Read the model definition and answer for the solid it produces. Units are mm, in the model's axes. A direction names the side the tool comes from. Coordinates: 2 decimals unless noted, no trailing zeros. Loops run counter-clockwise (first coordinate to the right, second up) from the corner with the lowest first, then second, coordinate; pieces in that order, holes last.
from build123d import *

# Parameters (mm, degrees)
SALIENTE_EXTRUIR1_DEPTH = 3
SALIENTE_EXTRUIR2_DEPTH = 1
CROQUIS1_7_W            = 1.8
CROQUIS1_7_H            = 10
SALIENTE_EXTRUIR4_DEPTH = 9.5
REDONDEO2_R             = 5
CROQUIS3_R              = 1.5
CORTAR_EXTRUIR2_DEPTH   = 16


with BuildPart() as part:
    # Croquis1 → Saliente-Extruir1 (new, symmetric)
    with BuildSketch(Plane(origin=(0, 0, 0), x_dir=(1, 0, 0), z_dir=(0, 1, 0))):
        with BuildLine():
            Line((-1.861867424, 4.190006044), (10.856046359, 4.190006044))
            ThreePointArc((10.856046359, 4.190006044), (12.977366702, 3.311326387), (13.856046359, 1.190006044))
            Line((13.856046359, 1.190006044), (13.856046359, -78.809993956))
            Line((13.856046359, -78.809993956), (10.856046359, -78.809993956))
            ThreePointArc((10.856046359, -78.809993956), (8.734726015, -77.9313143), (7.856046359, -75.809993956))
            Line((7.856046359, -75.809993956), (7.856046359, -40.566421369))
            Line((7.856046359, -40.566421369), (-4.195556186, -3.47994934))
            ThreePointArc((-4.195556186, -3.47994934), (-5.870430721, 1.219660174), (-1.861867424, 4.190006044))
        make_face()
        with BuildLine():
            Line((-1.861867424, 2.6), (2.138132576, 2.6))
            ThreePointArc((2.138132576, 2.6), (4.738132576, 0), (2.138132576, -2.6))
            Line((2.138132576, -2.6), (-1.861867424, -2.6))
            ThreePointArc((-1.861867424, -2.6), (-4.461867424, 0), (-1.861867424, 2.6))
        make_face(mode=Mode.SUBTRACT)
        Polygon((0.241081645, -4.190006044), (7.856046359, -4.190006044), (7.856046359, -27.623584675), align=None, mode=Mode.SUBTRACT)
    extrude(amount=SALIENTE_EXTRUIR1_DEPTH, both=True)

    # Croquis1<3> → Saliente-Extruir2 (add, symmetric)
    with BuildSketch(Plane(origin=(0, 0, 0), x_dir=(1, 0, 0), z_dir=(0, 1, 0))):
        with BuildLine():
            ThreePointArc((-1.861867424, 2.6), (-3.700345055, 1.838477631), (-4.461867424, 0))
            ThreePointArc((-4.461867424, 0), (-3.700345055, -1.838477631), (-1.861867424, -2.6))
            Line((-1.861867424, -2.6), (2.138132576, -2.6))
            ThreePointArc((2.138132576, -2.6), (4.738132576, 0), (2.138132576, 2.6))
            Line((2.138132576, 2.6), (-1.861867424, 2.6))
        make_face()
        with BuildLine():
            ThreePointArc((-0.591867424, 0), (-1.861867424, -1.27), (-3.131867424, 0))
            ThreePointArc((-3.131867424, 0), (-1.861867424, 1.27), (-0.591867424, 0))
        make_face(mode=Mode.SUBTRACT)
        with BuildLine():
            ThreePointArc((3.408132576, 0), (2.138132576, -1.27), (0.868132576, 0))
            ThreePointArc((0.868132576, 0), (2.138132576, 1.27), (3.408132576, 0))
        make_face(mode=Mode.SUBTRACT)
    extrude(amount=SALIENTE_EXTRUIR2_DEPTH, both=True)

    # Croquis1<7> → Saliente-Extruir4 (add, symmetric)
    with BuildSketch(Plane(origin=(0, 0, 0), x_dir=(1, 0, 0), z_dir=(0, 1, 0))):
        with Locations((12.956046359, -9.190006044)):
            Rectangle(CROQUIS1_7_W, CROQUIS1_7_H)
        with Locations((12.956046359, -69.190006044)):
            Rectangle(CROQUIS1_7_W, CROQUIS1_7_H)
    extrude(amount=SALIENTE_EXTRUIR4_DEPTH, both=True)

    # Redondeo2
    # the kernel refuses this fillet: 5 mm, written as the material it takes off along each edge
    with BuildSketch(Plane(origin=(-0.443953641, -9.5, 74.190006044), x_dir=(0, 1, 0), z_dir=(1, 0, 0)), Plane(origin=(26.356046359, -9.5, 64.190006044), x_dir=(0, 1, 0), z_dir=(-1, 0, 0)), Plane(origin=(-0.443953641, -9.5, 14.190006044), x_dir=(0, 1, 0), z_dir=(1, 0, 0)), Plane(origin=(26.356046359, -9.5, 4.190006044), x_dir=(0, 1, 0), z_dir=(-1, 0, 0))) as redondeo2_piece_1:
        with BuildLine():
            CenterArc((REDONDEO2_R, -REDONDEO2_R), REDONDEO2_R, 90, 90)
            Line((0, -REDONDEO2_R), (-REDONDEO2_R * 0.02, -REDONDEO2_R))
            Line((-REDONDEO2_R * 0.02, -REDONDEO2_R), (-REDONDEO2_R * 0.02, REDONDEO2_R * 0.02))
            Line((-REDONDEO2_R * 0.02, REDONDEO2_R * 0.02), (REDONDEO2_R, REDONDEO2_R * 0.02))
            Line((REDONDEO2_R, REDONDEO2_R * 0.02), (REDONDEO2_R, 0))
        make_face()
    extrude(amount=26.8, mode=Mode.SUBTRACT)
    with BuildSketch(Plane(origin=(-0.443953641, 9.5, 74.190006044), x_dir=(0, -1, 0), z_dir=(1, 0, 0)), Plane(origin=(26.356046359, 9.5, 64.190006044), x_dir=(0, -1, 0), z_dir=(-1, 0, 0)), Plane(origin=(-0.443953641, 9.5, 14.190006044), x_dir=(0, -1, 0), z_dir=(1, 0, 0)), Plane(origin=(26.356046359, 9.5, 4.190006044), x_dir=(0, -1, 0), z_dir=(-1, 0, 0))) as redondeo2_piece_2:
        with BuildLine():
            CenterArc((REDONDEO2_R, REDONDEO2_R), REDONDEO2_R, 180, 90)
            Line((0, REDONDEO2_R), (-REDONDEO2_R * 0.02, REDONDEO2_R))
            Line((-REDONDEO2_R * 0.02, REDONDEO2_R), (-REDONDEO2_R * 0.02, -REDONDEO2_R * 0.02))
            Line((-REDONDEO2_R * 0.02, -REDONDEO2_R * 0.02), (REDONDEO2_R, -REDONDEO2_R * 0.02))
            Line((REDONDEO2_R, -REDONDEO2_R * 0.02), (REDONDEO2_R, 0))
        make_face()
    extrude(amount=26.8, mode=Mode.SUBTRACT)

    # Croquis3 → Cortar-Extruir2 (cut)
    with BuildSketch(Plane(origin=(13.856046359, 0, 0), x_dir=(0, 0, -1), z_dir=(1, 0, 0))):
        with Locations((-69.190006044, 7.5)):
            Circle(CROQUIS3_R)
        with Locations((-69.190006044, -7.5)):
            Circle(CROQUIS3_R)
        with Locations((-9.190006044, 7.5)):
            Circle(CROQUIS3_R)
        with Locations((-9.190006044, -7.5)):
            Circle(CROQUIS3_R)
    extrude(amount=-CORTAR_EXTRUIR2_DEPTH, mode=Mode.SUBTRACT)


solid = part.part
Item 1: A cutting plane is placed at C-C on y = 2. Determine the outline of the cut face in (x, z), then the cut area to 3 significant figures.
Numbers:
outline: (-4.2, 3.48) arc R4.19 ccw to (-1.86, -4.19) - (10.86, -4.19) arc R3 ccw to (13.86, -1.19) - (13.86, 78.81) - (10.86, 78.81) arc R3 ccw to (7.86, 75.81) - (7.86, 40.57) - close; hole (-1.86, -2.6) - (2.14, -2.6) arc R2.6 ccw to (2.14, 2.6) - (-1.86, 2.6) arc R2.6 ccw to start; hole (0.24, 4.19) - (7.86, 4.19) - (7.86, 27.62) - close
area: 687 mm2
Item 2: Which of the six approach directions +Z, -Z, +X, -X, +Y, -Y give full straight-line access (tool end or side, diameter ignored) to faces 5 (the face through (4, 0, 4.19)), 6 (the face through (4.738, 2.014, -0.057)), 7 (the face through (13, -4, 4.19)), 8 (the face through (4.738, -1.986, -0.057))?
Numbers:
face 5: +Y, -Y
face 6: +Y
face 7: -Z, +X, -X, -Y
face 8: -Y
Item 3: A cutting plane is placed at A-A on z = 0. Determine the outline of the cut face in (x, y).
Numbers:
outline: (-6.05, -3) - (-4.46, -3) - (-4.46, -1) - (-3.13, -1) - (-3.13, 1) - (-4.46, 1) - (-4.46, 3) - (-6.05, 3) - close; (-0.59, -1) - (0.87, -1) - (0.87, 1) - (-0.59, 1) - close; (3.41, -1) - (4.74, -1) - (4.74, -3) - (13.86, -3) - (13.86, 3) - (4.74, 3) - (4.74, 1) - (3.41, 1) - close
Item 4: A cutting plane is placed at B-B on y = -7.5. Determine the outline of the cut face in (x, z).
Numbers:
outline: (12.06, 5.19) - (13.86, 5.19) - (13.86, 7.69) - (12.06, 7.69) - close; (12.06, 10.69) - (13.86, 10.69) - (13.86, 13.19) - (12.06, 13.19) - close; (12.06, 65.19) - (13.86, 65.19) - (13.86, 67.69) - (12.06, 67.69) - close; (12.06, 70.69) - (13.86, 70.69) - (13.86, 73.19) - (12.06, 73.19) - close
Item 5: Determine the mould class of faces 1 (the face through (13, 4, 14.19)), 2 (the face through (12.97, -8.41, 70.38)), 3 (the face through (12.9, 9.5, 9.1)), 4 (the face through (13, -9.5, 69.1)) for opening direction Y: released by +Y, released by -Y, zero draft, split by the parting line, or undercut.
Numbers:
face 1: zero draft
face 2: undercut
face 3: released by +Y
face 4: released by -Y
Item 6: Find the intervals of material crossed by line 1 along Y through (x, z) = (3.5, 19.5); line 2 along Z through (x, y) = (12.25, -3.5); line 3 along X through (y, z) = (-6, 12.5), in increasing order.
Numbers:
line 1: y = -3 to 3
line 2: z = 4.19 to 14.19, 64.19 to 74.19
line 3: x = 12.06 to 13.86
Item 7: A cutting plane is placed at D-D on z = 24. Determine the outline of the cut face in (x, y), then the cut area to 3 significant figures.
Numbers:
outline: (2.47, -3) - (6.68, -3) - (6.68, 3) - (2.47, 3) - close; (7.86, -3) - (13.86, -3) - (13.86, 3) - (7.86, 3) - close
area: 61.2 mm2
Item 8: Given pin 1 (0.8 mm diameter, centred on x = 13.5, y = 4, fed in from -Z); pin 2 (1 mm diameter, centred on x = 10.5, z = 21, fed in from +Y); pin 3 (6 mm diameter, centred on y = 5.5, z = 62.5, fed in from -X); pin 4 (2.5 mm diameter, centred on y = 7.5, z = 9.19, fed in from +X), each flat-ended and moving along its own axis, determine where each tip first touches the part or whether it passes through.
Numbers:
pin 1: stops at z = 4.19
pin 2: stops at y = 3
pin 3: stops at x = 7.86
pin 4: passes through
